Could you check a few things on this model? Use its own coordinates, in mm. A direction names the side the tool comes from. Give positions to 0.01 mm unless a question says otherwise; leave off trailing zeros. Write each loop counter-clockwise with the first axis right and the second up, starting at its lowest first coordinate (ties: lowest second). Pieces come first, ordered by that corner, then holes. Notation, with made-up numbers: (86, -27.5) - (111, -27.5) arc R30 cw to (111, 10.5) - close; hole circle Ø5 at (55, 9.5). An arc over 180 degrees is marked (long way). Answer in a Markdown table with one row per item.
from build123d import *

# Parameters (mm, degrees)
F2_R          = 1.5
F3_DEPTH      = 27.001
F4_R          = 3
F4_R_2        = 1.5
F5_DEPTH      = 7
F6_W          = 1
F6_H          = 45
F7_DEPTH      = 7
F7_DEPTH_BACK = 25
F8_R          = 1.25
F9_DEPTH      = 27.001
F10_R         = 1.6
F10_R_2       = 1.25
F11_DEPTH     = 5


with BuildPart() as f1:
    # F0 (on Top) → F1 (revolve)
    with BuildSketch(Plane.XY):
        Polygon((0, 15), (0, 4.25), (27, 4.25), (27, 7), (12, 7), (12, 15), align=None)
    revolve(axis=Axis((49.570793286, 0, 0), (1, 0, 0)))

    # F2 (on face) → F3 (cut, through all)
    with BuildSketch(Plane(origin=(0, 0, 0), x_dir=(0, -1, 0), z_dir=(-1, 0, 0))):
        with Locations((5.5, 9.5262794416)):
            Circle(F2_R)
        with Locations((-11, 0)):
            Circle(F2_R)
        with Locations((5.5, -9.5262794416)):
            Circle(F2_R)
    extrude(amount=-F3_DEPTH, mode=Mode.SUBTRACT)

    # F4 (on face) → F5 (cut)
    with BuildSketch(Plane(origin=(0, 0, 0), x_dir=(0, -1, 0), z_dir=(-1, 0, 0))):
        with Locations((5.5, 9.5262794416)):
            Circle(F4_R)
        with Locations((5.5, 9.5262794416)):
            Circle(F4_R_2, mode=Mode.SUBTRACT)
        with Locations((-11, 0)):
            Circle(F4_R)
        with Locations((-11, 0)):
            Circle(F4_R_2, mode=Mode.SUBTRACT)
        with Locations((5.5, -9.5262794416)):
            Circle(F4_R)
        with Locations((5.5, -9.5262794416)):
            Circle(F4_R_2, mode=Mode.SUBTRACT)
    extrude(amount=-F5_DEPTH, mode=Mode.SUBTRACT)

    # F6 (on Front) → F7 (cut, two sides)
    with BuildSketch(Plane.XZ) as f7_sk:
        with Locations((5.1783517702, 0)):
            Rectangle(F6_W, F6_H)
    extrude(amount=-F7_DEPTH, mode=Mode.SUBTRACT)
    extrude(f7_sk.sketch, amount=F7_DEPTH_BACK, mode=Mode.SUBTRACT)

    # F8 (on face) → F9 (cut, through all)
    with BuildSketch(Plane(origin=(0, 0, 0), x_dir=(0, -1, 0), z_dir=(-1, 0, 0))):
        with Locations((10, 0)):
            Circle(F8_R)
    extrude(amount=-F9_DEPTH, mode=Mode.SUBTRACT)

    # F10 (on face) → F11 (cut)
    with BuildSketch(Plane(origin=(0, 0, 0), x_dir=(0, -1, 0), z_dir=(-1, 0, 0))):
        with Locations((10, 0)):
            Circle(F10_R)
        with Locations((10, 0)):
            Circle(F10_R_2, mode=Mode.SUBTRACT)
    extrude(amount=-F11_DEPTH, mode=Mode.SUBTRACT)


solid = f1.part
1) Imagine slicing it at C-C (y = 11). List the corners of the cut face in (x, z) for me.
Check values:
| item | result |
|---|---|
| outline | (0, -10.2) - (12, -10.2) - (12, -1.5) - (7, -1.5) - (7, -3) - (0, -3) - close; (0, 3) - (7, 3) - (7, 1.5) - (12, 1.5) - (12, 10.2) - (0, 10.2) - close |
2) On a 3-axis mill with a long thin cutter (end or side, diameter ignored), from which of +Z, -Z, +X, -X, +Y, -Y can I reach the whole of each face in a straight line? I mean faces 4 (the face through (4.678, -4, 3)), 5 (the face through (12, -3.1, -6.5)), 6 (the face through (2.31, -5.11, -6.55)). Say none if no direction works.
Check values:
| item | result |
|---|---|
| face 4 | +Z, -Z, -Y |
| face 5 | +X |
| face 6 | -X |
3) We'd pull the mould along Y, two halves only. Please class faces 1 (the face through (5, 7, 0)), 2 (the face through (7, -7, -11)), 3 (the face through (19.395, 6.466, -2.681)): +Y half, -Y half, draft (parallel to the pull), parting line (faces both ways), or undercut.
Check values:
| item | result |
|---|---|
| face 1 | -Y half |
| face 2 | undercut |
| face 3 | parting line |
4) Will these pins go through, and if not, where does the flat tip stop? P1, Ø3, axis at y = -10, z = 0, coming from the -X side; P2, Ø2.5, axis at y = -5.5, z = 9.53, coming from the +X side; P3, Ø12, axis at y = 11, z = 12, coming from the +X side; P4, Ø12, axis at x = 5, y = -7.5, coming from the -Z side.
Check values:
| item | result |
|---|---|
| P1 | stops at x = 5.68 |
| P2 | passes through |
| P3 | stops at x = 12 |
| P4 | stops at z = -14.92 |
5) If I drill on line 1 (X direction, y = -9.5, z = 5.75); line 2 (Y direction, x = 15.75, z = -0.25); line 3 (X direction, y = -8, z = -11), over which ranges is the centre line in solid material (lowest first)?
Check values:
| item | result |
|---|---|
| line 1 | x = 0 to 4.68, 5.68 to 12 |
| line 2 | y = -7 to -4.24, 4.24 to 7 |
| line 3 | x = 7 to 12 |
6) Imagine slicing it at B-B (z = 12). List the corners of the cut face in (x, y) for me.
Check values:
| item | result |
|---|---|
| outline | (0, -9) - (4.68, -9) - (4.68, -7.2) - (0, -7.2) - close; (0, -3.8) - (4.68, -3.8) - (4.68, 7) - (5.68, 7) - (5.68, -3.8) - (7, -3.8) - (7, -7.2) - (5.68, -7.2) - (5.68, -9) - (12, -9) - (12, 9) - (0, 9) - close |
7) Imagine slicing it at D-D (z = 0). State how many separate pieces and enclosed holes the cut face has, then the cut area to 3 significant figures.
Check values:
| item | result |
|---|---|
| separate pieces | 6 |
| enclosed holes | 0 |
| area | 239 mm2 |
8) Imagine slicing it at A-A (y = 0). List the corners of the cut face in (x, z) for me, then the cut area to 3 significant figures.
Check values:
| item | result |
|---|---|
| outline | (0, -15) - (4.68, -15) - (4.68, -4.25) - (0, -4.25) - close; (0, 4.25) - (4.68, 4.25) - (4.68, 15) - (0, 15) - close; (5.68, -15) - (12, -15) - (12, -7) - (27, -7) - (27, -4.25) - (5.68, -4.25) - close; (5.68, 4.25) - (27, 4.25) - (27, 7) - (12, 7) - (12, 15) - (5.68, 15) - close |
| area | 319 mm2 |
